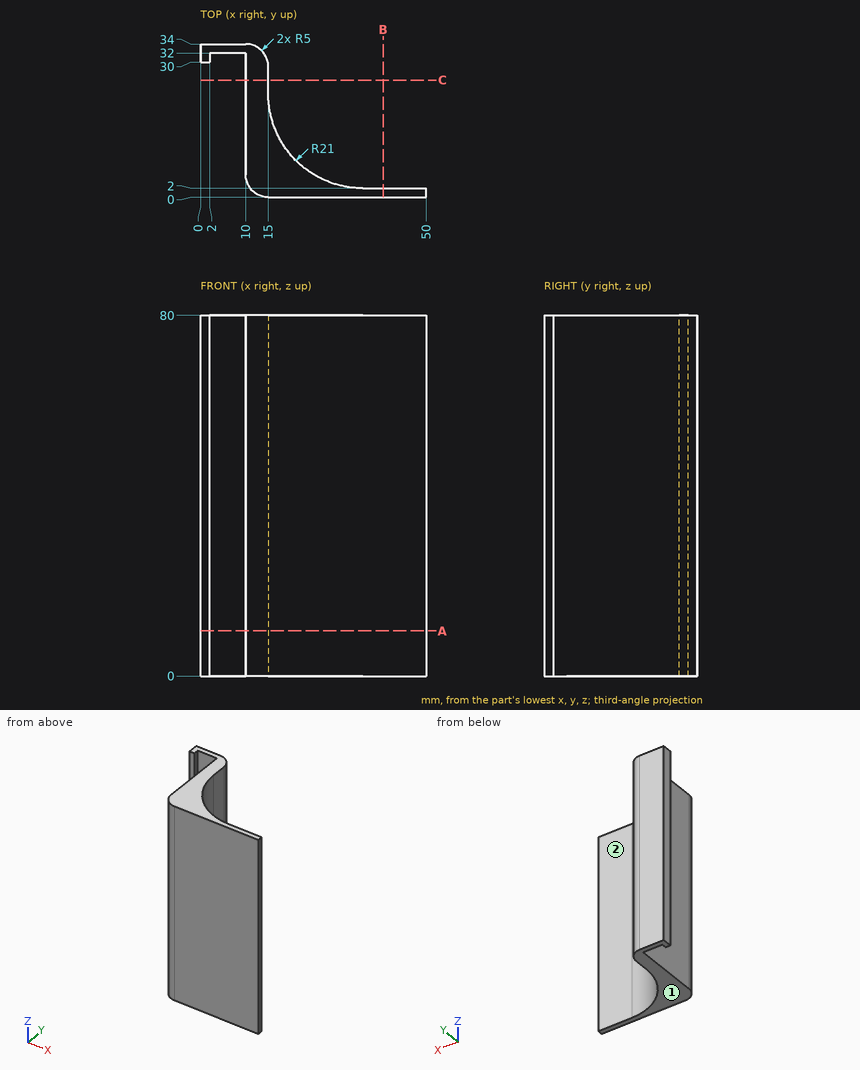
Here's the drawing with two shaded views (mm, measured from the low corner). I have some questions. A direction names the side the tool comes from. Give positions to 0.01 mm unless a question says otherwise; leave off trailing zeros. Loops run counter-clockwise (first coordinate to the right, second up) from the corner with the lowest first, then second, coordinate; pieces in that order, holes last. Notation, with made-up numbers: M -6.5,45 L 27.5,45 A25 ccw 27.5,62 Z; hole C 33,-13 d5. An arc over 180 degrees is marked long. Use one line per item in the form item = value. Start each with the question number.
Q1. Will these pins go through, and if not, where does the flat tip stop? pin 1 Ø1 at (x, z) = (1.5, 33) entering from -Y; pin 2 Ø7 at (x, z) = (40.5, 45.5) entering from +Y; pin 3 Ø12 at (y, z) = (6.5, 16) entering from -X.
Q2. If we section it at C-C (y = 26): Write out the boundary of the cut face in (x, z), then the cut area to 3 significant figures.
Q3. I need wall thicknesses on line 1 along Y through (x, z) = (43, 66); line 2 along Y through (x, z) = (3, 12); line 3 along X through (y, z) = (15, 21.5). Which ranges of each line are inside material? Lowest first, please.
Q4. If we section it at B-B (x = 40.5): Write out the boundary of the cut face in (y, z), then the cut area to 3 significant figures.
Q5. Which directions (+Z, -Z, +X, -X, +Y, -Y) give clear straight access to the entire face, cutting with the end or side of a thin tool? Please do the marked faces 1 and 2.
Q6. If we section it at A-A (z = 10): Write out the boundary of the cut face in (x, y).
Taken from the geometry:
q1.pin_1 = 30
q1.pin_2 = 2
q1.pin_3 = 10
q2.outline = M 10,0 L 15,0 L 15,80 L 10,80 Z
q2.area = 400 mm^2
q3.line_1 = 0 to 2
q3.line_2 = 32 to 34
q3.line_3 = 10 to 16.58
q4.outline = M 0,0 L 2,0 L 2,80 L 0,80 Z
q4.area = 160 mm^2
q5.face_1 = -Z, +X, -X, +Y, -Y
q5.face_2 = +Z, -Z, +X, +Y
q6.outline = M 0,30 L 2,30 L 2,32 L 10,32 L 10,5 A5 ccw 15,0 L 50,0 L 50,2 L 36,2 A21 cw 15,23 L 15,29 A5 ccw 10,34 L 0,34 Z
